Can you work these out from the model? Positions are in its coordinate system, mm. A direction names the side the tool comes from. Coordinates: 2 decimals unless noted, no trailing zeros. Write each loop counter-clockwise with the first axis right and the second up, starting at its lowest first coordinate (ties: lowest second). Pieces come first, ordered by that corner, then holes. Notation, with made-up numbers: (-20, 50) -> (-6, 50) arc R15 cw to (-6, 54) -> close; hole circle Ø7 at (76.25, 53.5). An arc over 180 degrees is marked (long way). Answer as CSV lines item,"result". Start each with the question number.
```python
from build123d import *

# Parameters (mm, degrees)
ESQUISSE2_R        = 2.1
BOSS_EXTRU_2_DEPTH = 5


with BuildPart() as part:
    # Esquisse2 → Boss.-Extru.2 (new body)
    with BuildSketch(Plane(origin=(0, 0, 0), x_dir=(0, 0, -1), z_dir=(1, 0, 0))):
        with BuildLine():
            Line((7.750863413, -22.545340393), (12.249833074, -22.545340393))
            ThreePointArc((12.249833074, -22.545340393), (12.676550763, -22.722176075), (12.499999941, -22.295340449))
            Line((12.499999941, -22.295340449), (12.499999941, -17.045209493))
            ThreePointArc((12.499999941, -17.045209493), (12.646553376, -16.691549218), (13.000302135, -16.545209493))
            Line((13.000302135, -16.545209493), (17.000089808, -16.545209493))
            ThreePointArc((17.000089808, -16.545209493), (17.353706499, -16.69180921), (17.499999941, -17.04555272))
            Line((17.499999941, -17.04555272), (17.499999941, -25.545209493))
            ThreePointArc((17.499999941, -25.545209493), (16.9143288, -26.959538351), (15.499999941, -27.545209493))
            Line((15.499999941, -27.545209493), (-15.500000059, -27.545209493))
            ThreePointArc((-15.500000059, -27.545209493), (-16.914213621, -26.959423055), (-17.500000059, -25.545209493))
            Line((-17.500000059, -25.545209493), (-17.500000059, -17.04542182))
            ThreePointArc((-17.500000059, -17.04542182), (-17.35349126, -16.691718292), (-16.999787732, -16.545209493))
            Line((-16.999787732, -16.545209493), (-13.000000059, -16.545209493))
            ThreePointArc((-13.000000059, -16.545209493), (-12.646446668, -16.691656102), (-12.500000059, -17.045209493))
            Line((-12.500000059, -17.045209493), (-12.500000059, -22.295209493))
            ThreePointArc((-12.500000059, -22.295209493), (-12.676776754, -22.721986188), (-12.250000059, -22.545209493))
            Line((-12.250000059, -22.545209493), (-7.750394504, -22.545209493))
            ThreePointArc((-7.750394504, -22.545209493), (-7.32375732, -22.722125589), (-7.500000059, -22.295209803))
            Line((-7.500000059, -22.295209803), (-7.500000059, 18.204252682))
            ThreePointArc((-7.500000059, 18.204252682), (-7.322400285, 18.631591193), (-7.750017362, 18.454663189))
            Line((-7.750017362, 18.454663189), (-15.500000059, 18.454663189))
            ThreePointArc((-15.500000059, 18.454663189), (-16.914213621, 19.040449627), (-17.500000059, 20.454663189))
            Line((-17.500000059, 20.454663189), (-17.500000059, 28.954790507))
            ThreePointArc((-17.500000059, 28.954790507), (-17.353414349, 29.308483098), (-16.999606545, 29.454790507))
            Line((-16.999606545, 29.454790507), (-12.999606545, 29.454790507))
            ThreePointArc((-12.999606545, 29.454790507), (-12.646446514, 29.308344052), (-12.500000059, 28.955184021))
            Line((-12.500000059, 28.955184021), (-12.500000059, 23.705183903))
            ThreePointArc((-12.500000059, 23.705183903), (-12.676711319, 23.278492956), (-12.249849272, 23.454790507))
            Line((-12.249849272, 23.454790507), (-7.749606545, 23.454790507))
            ThreePointArc((-7.749606545, 23.454790507), (-7.322690777, 23.278152995), (-7.500000059, 23.704790197))
            Line((-7.500000059, 23.704790197), (-7.500000059, 30.955184021))
            ThreePointArc((-7.500000059, 30.955184021), (-7.353221822, 31.308675666), (-6.999455449, 31.454790507))
            Line((-6.999455449, 31.454790507), (6.999757524, 31.454790507))
            ThreePointArc((6.999757524, 31.454790507), (7.353328546, 31.308568754), (7.499999941, 30.955184021))
            Line((7.499999941, 30.955184021), (7.499999941, 23.704790197))
            ThreePointArc((7.499999941, 23.704790197), (7.323085388, 23.277909123), (7.749756946, 23.455328378))
            Line((7.749756946, 23.455328378), (12.250151348, 23.455328378))
            ThreePointArc((12.250151348, 23.455328378), (12.677119893, 23.279136755), (12.499999941, 23.705721037))
            Line((12.499999941, 23.705721037), (12.499999941, 28.955721891))
            ThreePointArc((12.499999941, 28.955721891), (12.646778178, 29.309213536), (13.00054455, 29.455328378))
            Line((13.00054455, 29.455328378), (17.00054455, 29.455328378))
            ThreePointArc((17.00054455, 29.455328378), (17.353745932, 29.308689359), (17.499999941, 28.955328378))
            Line((17.499999941, 28.955328378), (17.499999941, 20.454659607))
            ThreePointArc((17.499999941, 20.454659607), (16.914406065, 19.040638558), (15.50054455, 18.454659607))
            Line((15.50054455, 18.454659607), (7.75039284, 18.454659607))
            ThreePointArc((7.75039284, 18.454659607), (7.323611584, 18.631024058), (7.499999941, 18.204252682))
            Line((7.499999941, 18.204252682), (7.499999941, -22.295209803))
            ThreePointArc((7.499999941, -22.295209803), (7.32434554, -22.722243416), (7.750863413, -22.545340393))
        make_face()
        with Locations((-5.9e-08, 1.954659607)):
            Circle(ESQUISSE2_R, mode=Mode.SUBTRACT)
    extrude(amount=BOSS_EXTRU_2_DEPTH)


solid = part.part
```
Q1. I need wall thicknesses on L1, parallel to Z at x = 2.4, y = 28.5; L2, parallel to Z at x = 2.8, y = 23.5; L3, parallel to Y at x = 1.7, z = -11. Which ranges of each line are inside material? Lowest first, please.
Q2. Imagine slicing it at B-B (y = -19). Write out the boundary of the cut face in (x, z), then the cut area to 3 significant figures.
Q3. If we mould it in two halves opening along Y, with no side actions, what happens to faces 1 (the face through (2, -2, -7.5)), 2 (the face through (2, 27, 7.5)), 3 (the face through (2, 23.455, -10))? For each: released by +Y, released by -Y, zero draft, split by the parting line, or undercut.
Q4. Imagine slicing it at C-C (z = -11.5). Write out the boundary of the cut face in (x, y).
Q5. Which directions (+Z, -Z, +X, -X, +Y, -Y) give clear straight access to the entire face, cutting with the end or side of a thin tool? Please do faces 4 (the face through (2, 29.455, 15)), 5 (the face through (2, 18.455, 12)), 6 (the face through (2, -22.545, -10)).
Q6. Imagine slicing it at A-A (z = 0). Write out the boundary of the cut face in (x, y), then the cut area to 3 significant figures.
Q7. For pin 1 (1 mm diameter, centred on x = 3.5, y = -9.5, fed in from -Z); pin 2 (2 mm diameter, centred on x = 1.5, z = -15.5, fed in from +Y); pin 3 (1.5 mm diameter, centred on x = 4, y = 6, fed in from +Z), each with a flat end and sliding along its axis, tell me the tip position at first contact or that it passes through.
Entries:
1,L1,"-17.5 to -12.5, -7.5 to 7.5, 12.5 to 17.5"
1,L2,"-17.5 to -12.75, -7.25 to 7.25, 12.75 to 17.5"
1,L3,"-27.55 to -22.55, 18.45 to 23.46"
2,outline,"(0, -17.5) -> (5, -17.5) -> (5, -12.5) -> (0, -12.5) -> close; (0, -7.5) -> (5, -7.5) -> (5, 7.5) -> (0, 7.5) -> close; (0, 12.5) -> (5, 12.5) -> (5, 17.5) -> (0, 17.5) -> close"
2,area,"125 mm2"
3,face 1,"undercut"
3,face 2,"zero draft"
3,face 3,"released by +Y"
4,outline,"(0, -27.55) -> (5, -27.55) -> (5, -22.55) -> (0, -22.55) -> close; (0, 18.45) -> (5, 18.45) -> (5, 23.46) -> (0, 23.46) -> close"
5,face 4,"+Z, +X, -X, +Y"
5,face 5,"+Z, +X, -X"
5,face 6,"+X, -X"
6,outline,"(0, -27.55) -> (5, -27.55) -> (5, -0.15) -> (0, -0.15) -> close; (0, 4.05) -> (5, 4.05) -> (5, 31.45) -> (0, 31.45) -> close"
6,area,"274 mm2"
7,pin 1,"z = -7.5"
7,pin 2,"y = 29.46"
7,pin 3,"z = 7.5"
